```python
from build123d import *

# Parameters (mm, degrees)
F0_R     = 25
F1_DEPTH = 10
F2_R     = 5


with BuildPart() as f1:
    # F0 (on Top) → F1 (new body, symmetric)
    with BuildSketch(Plane.XY):
        Circle(F0_R)
    extrude(amount=F1_DEPTH, both=True)

    # F2
    f2_edges = [f1.edges().sort_by_distance(p)[0] for p in [
        (-25, 0, 10),
    ]]
    fillet(f2_edges, radius=F2_R)

    # F3: F1 across face


with BuildPart() as f1_1:
    add(f1.part)
    add(f1.part.mirror(Plane.XY.offset(10)))


solid = f1_1.part
```
CAD build for the part. Positions are in the model's coordinates, mm. Coordinates: 2 decimals unless noted, no trailing zeros. Order: outer loops, then holes, each group sorted by start corner. A loop starts at its lowest first (then second) coordinate and runs counter-clockwise, first axis right, second up. Notation, with made-up numbers: (-11.5, 85.5) -> (15.5, 85.5) arc R27 cw to (15.5, 124.5) -> close; hole circle Ø8 at (36.5, 2). An arc over 180 degrees is marked (long way). Use one line per item in the form item = value. Start each with the question number.
1) Drill centre lines: L1, parallel to Y at x = -0.5, z = 6.5; L2, parallel to X at y = -4.5, z = 8; L3, parallel to X at y = -9.5, z = 28.5. Where is each one in solid material? Low to high. Write a range as [from, to].
2) Drop flat-ended pins along their axis: pin 1 (1.5 mm diameter, centred on y = -9.5, z = 20.5, fed in from +X); pin 2 (8 mm diameter, centred on x = 9, z = 8.5, fed in from +Y); pin 3 (10 mm diameter, centred on y = 13.5, z = 13.5, fed in from -X). Give the stop position or say it passes through.
3) Band-saw the part on A-A on z = 21. Give the cut face in (x, y).
4) Band-saw the part on B-B on z = 11.5. Give the cut face in (x, y).
Entries:
q1.L1 = [-24.76, 24.76]
q1.L2 = [-23.57, 23.57]
q1.L3 = [-23.12, 23.12]
q2.pin_1 = 23.42
q2.pin_2 = 24.2
q2.pin_3 = -23.45
q3.outline = circle Ø50 at (0, 0)
q4.outline = circle Ø47.14 at (0, 0)
